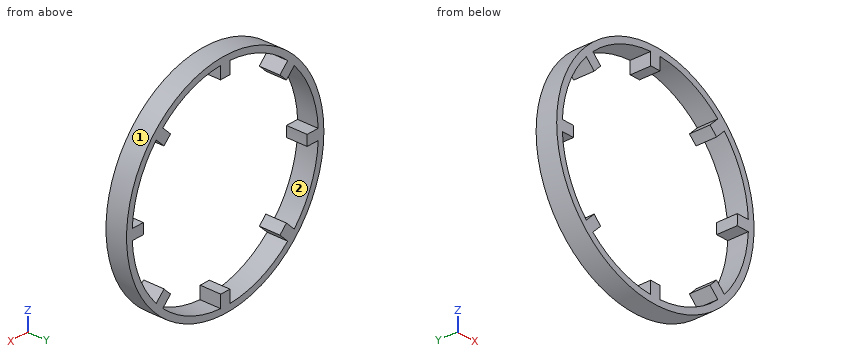
Autodesk Inventor part; units mm, degrees
ref_plane "YZ Plane" through (0, 0, 0) normal (1, 0, 0) x (0, 1, 0)
ref_plane "XZ Plane" through (0, 0, 0) normal (0, 1, 0) x (-1, 0, 0)
ref_plane "XY Plane" through (0, 0, 0) normal (0, 0, 1) x (1, 0, 0)
sketch "Sketch1" plane through (0, 0, 0) normal (0, 1, 0) x (-1, 0, 0)
  circle A0 centre (0, 0) radius 43.28 construction
  circle A1 centre (0, 0) radius 44.28
  circle A2 centre (0, 0) radius 50.28
  circle A3 centre (0, 0) radius 53.28
  line L0 (2.5, -53.28) -> (-2.5, -53.28)
  line L1 (-2.5, -53.28) -> (-2.5, 0)
  line L2 (-2.5, 0) -> (2.5, 0)
  line L3 (2.5, 0) -> (2.5, -53.28)
  point P0 (0, -53.28)
  point P1 (-2.5, -50.2178)
  point P2 (2.5, -50.2178)
  point P3 (2.5, -44.2094)
  point P4 (-2.5, -44.2094)
  dimension "d0" = 86.56
  dimension "d1" = 1
  dimension "d2" = 6
  dimension "d3" = 3
  dimension "d4" = 5
extrude "Extrusion1" add sketch "Sketch1" along normal blind 10 contours L1 A3 L3 A2 | A2 L3 A3 L1
extrude "Extrusion2" add sketch "Sketch1" along normal blind 10 contours A1 L3 A2 L1 picked at (-1.9446, -46.2331)
pattern_circular "Circular Pattern1" count 8 over 360 about axis through (0, -10, 0) along (0, 1, 0) of "Extrusion2"
properties part number "STI Hybrid 98 Cooling Shroud Upper Section Prototype_3DPrint"
Design review of the part built by this model. Coordinates are the model's own, in mm. Face numbers are marked on the shaded views. Give positions to 0.01 mm unless a question says otherwise; leave off trailing zeros. Write each loop counter-clockwise with the first axis right and the second up, starting at its lowest first coordinate (ties: lowest second). Pieces come first, ordered by that corner, then holes. Notation, with made-up numbers: M -6.5,30 L 11.5,30 A6 ccw 11.5,39 Z; hole C 69.5,-9.5 d1. An arc over 180 degrees is marked long. Return JSON: item names as keys, results as strings. Group by question number.
Item 1: The part is to be moulded in two halves that separate along Z. For the marked faces 1 and 2, say which applies: pulls with the +Z half, pulls with the -Z half, needs draft (parallel to the pull), parting line crosses it, or undercut.
Item 2: Wall thickness on line 1 along Z through (x, y) = (1, 9.5); line 2 along Z through (x, y) = (45.5, 8.5); line 3 along X through (y, z) = (8.5, -31.5): over which ranges is each line inside the solid? List them lowest first.
Item 3: Take a section at A-A (x = 0). Give the boundary of the cut face in (y, z), plus the area to 3 significant figures.
Item 4: Clearance check with flat-ended pins moving along their axes: pin 1 Ø1.8 at (x, y) = (47, 3.5) entering from -Z; pin 2 Ø5 at (y, z) = (7, -47) entering from -X; pin 3 Ø1 at (y, z) = (9, 21.5) entering from +X. State where each tip first meets the part, or that it passes through.
Item 5: Take a section at C-C (z = 0). Give the boundary of the cut face in (x, y), plus the area to 3 significant figures.
Return value:
{
 "1": {"face 1": "parting line crosses it", "face 2": "undercut"},
 "2": {"line 1": "z = -53.27 to -44.27, 44.27 to 53.27", "line 2": "z = -27.72 to -21.4, -2.5 to 2.5, 21.4 to 27.72", "line 3": "x = -42.97 to -39.19, -35.04 to -31.12, 31.12 to 35.04, 39.19 to 42.97"},
 "3": {"outline": "M 0,-53.28 L 10,-53.28 L 10,-44.28 L 0,-44.28 Z; M 0,44.28 L 10,44.28 L 10,53.28 L 0,53.28 Z", "area": "180 mm2"},
 "4": {"pin 1": "stops at z = -26.71", "pin 2": "stops at x = -29.3", "pin 3": "stops at x = 48.97"},
 "5": {"outline": "M -53.28,0 L -44.28,0 L -44.28,10 L -53.28,10 Z; M 44.28,0 L 53.28,0 L 53.28,10 L 44.28,10 Z", "area": "180 mm2"}
}
